Design review of the part built by this model. Coordinates are the model's own, in mm. Face numbers are marked on the shaded views. Coordinates: 2 decimals unless noted, no trailing zeros. Write each loop counter-clockwise with the first axis right and the second up, starting at its lowest first coordinate (ties: lowest second). Pieces come first, ordered by that corner, then holes.
Q1. Add section D-D, the plane x = -8. Give the boundary of the cut face in (y, z).
Q2. The part is to be moulded in two halves that separate along Z. For the marked faces 1 and 2, say which applies: +Z half, -Z half, draft (parallel to the pull), parting line (faces both ways), or undercut.
Q3. Add section A-A, the plane y = 0. Give the boundary of the cut face in (x, z) (3 decimals).
Q4. Clearance check with flat-ended pins moving along their axes: pin 1 Ø3 at (x, z) = (-8, -5) entering from -Y; pin 2 Ø2 at (x, z) = (7, -1.5) entering from -Y; pin 3 Ø1 at (y, z) = (-3, -6.5) entering from -X. State where each tip first meets the part, or that it passes through.
Q5. Add section C-C, the plane x = 17. Give the boundary of the cut face in (y, z) (3 decimals).
Q6. To check wall thickness, follow probe 1 along Z at (x, y) = (-14.65, 0); probe 2 along Z at (x, y) = (12.75, 0) (3 decimals); probe 3 along Y at (x, z) = (18.5, -1.5). State the ranges of each line that lie inside material, in increasing order.
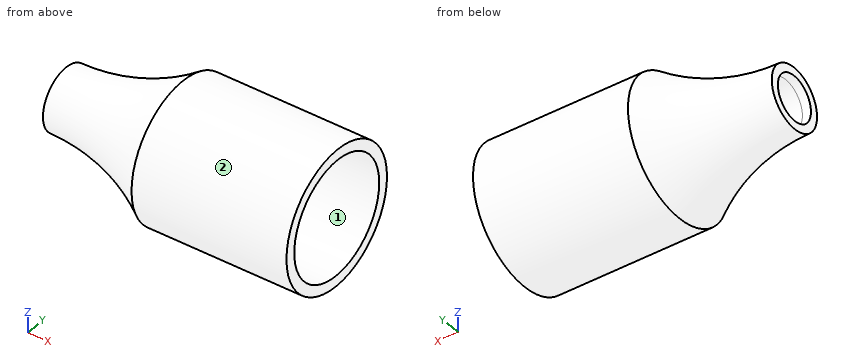
Autodesk Inventor part; units mm, degrees
ref_plane "YZ Plane" through (0, 0, 0) normal (1, 0, 0) x (0, 1, 0)
ref_plane "XZ Plane" through (0, 0, 0) normal (0, 1, 0) x (-1, 0, 0)
ref_plane "XY Plane" through (0, 0, 0) normal (0, 0, 1) x (1, 0, 0)
sketch "Sketch1" plane through (0, 0, 0) normal (1, 0, 0) x (0, 1, 0)
  circle A0 centre (0, 0) radius 7.5
  circle A1 centre (0, 0) radius 8.875
  dimension "d0" = 15
  dimension "d1" = 17.75
extrude "Extrusion1" add sketch "Sketch1" along normal blind 20
sketch "Sketch2" plane through (0, 0, 0) normal (0, 0, 1) x (1, 0, 0)
  line L0 (-15, 0) -> (-15, 4) construction
  arc A0 (-15, 4) -> (0, 8.875) centre (-15, 29.5144) ccw
  line L1 (-15, 4) -> (-2.0685, 4) construction
  arc A1 (-13.9, 2.9227) -> (0, 7.5297) centre (-15, 29.5144) ccw
  line L2 (-13.9, 2.9227) -> (-13.9, 0) construction
  line L3 (0, -8.875) -> (0, 8.875)
  line L4 (0, 8.875) -> (0, 7.5297)
  line L5 (-13.9, 2.9227) -> (-15, 2.9227)
  line L6 (-15, 2.9227) -> (-15, 4)
  line L7 (0, 0) -> (-13.9, 0) construction
  dimension "d4" = 15
  dimension "d6" = 4
  dimension "d7" = 1.1
revolve "Revolution1" add sketch "Sketch2" angle 360 about axis through (0, 0, 0) along (-1, 0, 0)
properties part number "5 mm nozle"
Here are the results:
1. outline: circle Ø9.96 at (0, 0); hole circle Ø7.67 at (0, 0)
2. face 1: undercut
2. face 2: parting line
3. outline: (-15, -4) arc R25.514 cw to (0, -8.875) - (20, -8.875) - (20, -7.5) - (0, -7.5) - (0, -7.53) arc R26.614 ccw to (-13.9, -2.923) - (-15, -2.923) - close; (-15, 2.923) - (-13.9, 2.923) arc R26.614 ccw to (0, 7.53) - (0, 7.5) - (20, 7.5) - (20, 8.875) - (0, 8.875) arc R25.514 cw to (-15, 4) - close
4. pin 1: stops at y = -3.67
4. pin 2: stops at y = -8.86
4. pin 3: stops at x = -3.66
5. outline: circle Ø17.75 at (0, 0); hole circle Ø15 at (0, 0)
6. probe 1: z = -4 to -2.92, 2.92 to 4
6. probe 2: z = -8.875 to -7.5, 7.5 to 8.875
6. probe 3: y = -8.75 to -7.35, 7.35 to 8.75
